```python
from build123d import *

# Parameters (mm, degrees)
SKETCH1_W           = 180
SKETCH1_H           = 150
SKETCH1_R           = 19
SKETCH1_R_2         = 2
SKETCH1_R_3         = 2.412227545
SKETCH1_R_4         = 2.29012976
SKETCH1_R_5         = 5
SKETCH1_R_6         = 3
BOSS_EXTRUDE3_DEPTH = 2.5
FILLET2_R           = 20
CUT_EXTRUDE1_REACH  = 4.5
SKETCH2_R           = 1.8


with BuildPart() as part:
    # Sketch1 → Boss-Extrude3 (new body)
    with BuildSketch(Plane.XY):
        with Locations((1.018867925, 17.603773585)):
            Rectangle(SKETCH1_W, SKETCH1_H)
        with Locations((-53.981132075, 42.603773585)):
            Circle(SKETCH1_R, mode=Mode.SUBTRACT)
        with Locations((-71.981132075, 63.603773585)):
            Circle(SKETCH1_R_2, mode=Mode.SUBTRACT)
        with Locations((-71.981132075, 21.603773585)):
            Circle(SKETCH1_R_2, mode=Mode.SUBTRACT)
        with Locations((-36.981132075, 63.603773585)):
            Circle(SKETCH1_R_3, mode=Mode.SUBTRACT)
        with Locations((-36.981132075, 21.603773585)):
            Circle(SKETCH1_R_4, mode=Mode.SUBTRACT)
        with Locations((39.018867925, 63.603773585)):
            Circle(SKETCH1_R_3, mode=Mode.SUBTRACT)
        with Locations((74.018867925, 63.603773585)):
            Circle(SKETCH1_R_2, mode=Mode.SUBTRACT)
        with Locations((74.018867925, 21.603773585)):
            Circle(SKETCH1_R_2, mode=Mode.SUBTRACT)
        with Locations((39.018867925, 21.603773585)):
            Circle(SKETCH1_R_4, mode=Mode.SUBTRACT)
        with Locations((56.018867925, 42.603773585)):
            Circle(SKETCH1_R, mode=Mode.SUBTRACT)
        with Locations((-37.797961742, -27.20701666)):
            Circle(SKETCH1_R_5, mode=Mode.SUBTRACT)
        with Locations((-37.797961742, -5.637572315)):
            Circle(SKETCH1_R_5, mode=Mode.SUBTRACT)
        with Locations((39.018867925, -5.760467761)):
            Circle(SKETCH1_R_5, mode=Mode.SUBTRACT)
        with Locations((1.018867925, -27.20701666)):
            Circle(SKETCH1_R_6, mode=Mode.SUBTRACT)
        with Locations((39.018867925, -27.20701666)):
            Circle(SKETCH1_R_5, mode=Mode.SUBTRACT)
        with Locations((56.018867925, 79.876860749)):
            Circle(SKETCH1_R_6, mode=Mode.SUBTRACT)
    extrude(amount=BOSS_EXTRUDE3_DEPTH)

    # Fillet2
    fillet2_edges = [part.edges().sort_by_distance(p)[0] for p in [
        (91.018867925, -57.396226415, 1.25),
        (-88.981132075, -57.396226415, 1.25),
        (-88.981132075, 92.603773585, 1.25),
        (91.018867925, 92.603773585, 1.25),
    ]]
    fillet(fillet2_edges, radius=FILLET2_R)

    # Sketch2 → Cut-Extrude1 (cut, up to next)
    with BuildSketch(Plane.XY.offset(2.5), mode=Mode.PRIVATE) as cut_extrude1_sk1:
        with Locations((-76.981132075, -45.396226415)):
            Circle(SKETCH2_R)
    cut_extrude1_tool1 = extrude(cut_extrude1_sk1.sketch, amount=-CUT_EXTRUDE1_REACH, mode=Mode.PRIVATE) & part.part
    add(cut_extrude1_tool1.solids().sort_by_distance((-76.981132, -45.396226, 2.5))[0], mode=Mode.SUBTRACT)
    # Sketch2 → Cut-Extrude1 (cut, up to next)
    with BuildSketch(Plane.XY.offset(2.5), mode=Mode.PRIVATE) as cut_extrude1_sk2:
        with Locations((79.018867925, -45.396226415)):
            Circle(SKETCH2_R)
    cut_extrude1_tool2 = extrude(cut_extrude1_sk2.sketch, amount=-CUT_EXTRUDE1_REACH, mode=Mode.PRIVATE) & part.part
    add(cut_extrude1_tool2.solids().sort_by_distance((79.018868, -45.396226, 2.5))[0], mode=Mode.SUBTRACT)
    # Sketch2 → Cut-Extrude1 (cut, up to next)
    with BuildSketch(Plane.XY.offset(2.5), mode=Mode.PRIVATE) as cut_extrude1_sk3:
        with Locations((-76.981132075, 80.603773585)):
            Circle(SKETCH2_R)
    cut_extrude1_tool3 = extrude(cut_extrude1_sk3.sketch, amount=-CUT_EXTRUDE1_REACH, mode=Mode.PRIVATE) & part.part
    add(cut_extrude1_tool3.solids().sort_by_distance((-76.981132, 80.603774, 2.5))[0], mode=Mode.SUBTRACT)
    # Sketch2 → Cut-Extrude1 (cut, up to next)
    with BuildSketch(Plane.XY.offset(2.5), mode=Mode.PRIVATE) as cut_extrude1_sk4:
        with Locations((79.018867925, 80.603773585)):
            Circle(SKETCH2_R)
    cut_extrude1_tool4 = extrude(cut_extrude1_sk4.sketch, amount=-CUT_EXTRUDE1_REACH, mode=Mode.PRIVATE) & part.part
    add(cut_extrude1_tool4.solids().sort_by_distance((79.018868, 80.603774, 2.5))[0], mode=Mode.SUBTRACT)


solid = part.part
```
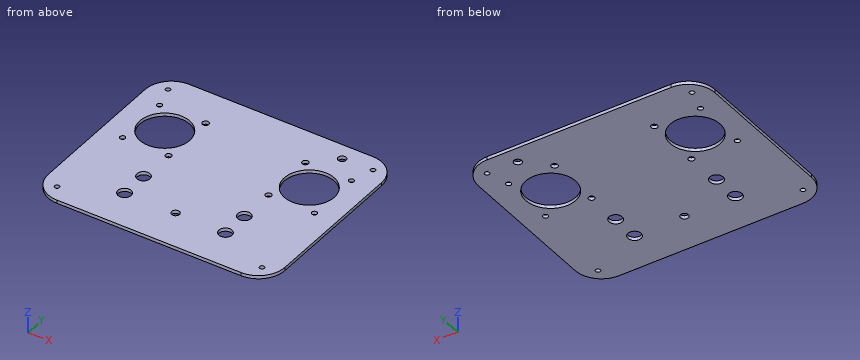
Source: CAD feature listing. Evaluate the final solid. Frame: model axes, mm. Coordinates: 2 decimals unless noted, no trailing zeros. Loops run counter-clockwise (first coordinate to the right, second up) from the corner with the lowest first, then second, coordinate; pieces in that order, holes last. Notation, with made-up numbers: (45.5, 8.25) -> (84.5, 8.25) arc R19 ccw to (84.5, 17.25) -> close; hole circle Ø7 at (89, 61). An arc over 180 degrees is marked (long way). One line per item, written item: value. Start each with the question number.
Q1. Section query A-A, the plane y = 34. Return the cut outline in (x, z).
Q2. Section query C-C, the plane z = 1.5. Give the number of separate pieces and of enclosed holes in the cut face, and give its area (3 significant figures).
Q3. Section query B-B, the plane x = 67. Return the cut outline in (y, z).
Q4. Line query: line 1 along X through (y, z) = (-45.5, 1.15); line 2 along X through (y, z) = (54, 1.95); line 3 along X through (y, z) = (-25, 0.65). Output: solid intervals per line, ascending.
Results:
1. outline: (-88.98, 0) -> (-70.92, 0) -> (-70.92, 2.5) -> (-88.98, 2.5) -> close; (-37.04, 0) -> (39.08, 0) -> (39.08, 2.5) -> (-37.04, 2.5) -> close; (72.96, 0) -> (91.02, 0) -> (91.02, 2.5) -> (72.96, 2.5) -> close
2. separate pieces: 1
2. enclosed holes: 20
2. area: 23,900 mm^2
3. outline: (-57.4, 0) -> (27.1, 0) -> (27.1, 2.5) -> (-57.4, 2.5) -> close; (58.11, 0) -> (92.6, 0) -> (92.6, 2.5) -> (58.11, 2.5) -> close
4. line 1: -87.27 to -78.78, -75.18 to 77.22, 80.82 to 89.3
4. line 2: -88.98 to -69.18, -38.78 to 40.82, 71.22 to 91.02
4. line 3: -88.98 to -42.28, -33.31 to -1.01, 3.05 to 34.53, 43.51 to 91.02
